Could you check a few things on this model? Use its own coordinates, in mm. A direction names the side the tool comes from. Coordinates: 2 decimals unless noted, no trailing zeros. Loops run counter-clockwise (first coordinate to the right, second up) from the corner with the lowest first, then second, coordinate; pieces in that order, holes last.
from build123d import *

# Parameters (mm, degrees)
F1_DEPTH = 25.4
F2_W     = 37.6737080514
F2_H     = 18.4638472274
F3_DEPTH = 101.6
F4_W     = 14.6301244386
F4_H     = 36.548535943
F5_DEPTH = 25.4
F6_DEPTH = 25.4
F7_W     = 18.4638472274
F7_H     = 37.6439765096
F8_DEPTH = 9.652


with BuildPart() as f1:
    # F0 (on Top) → F1 (new body)
    with BuildSketch(Plane.XY):
        with BuildLine():
            ThreePointArc((-18.8368540257, 0), (0, -18.8368540257), (18.8368540257, 0))
            Line((18.8368540257, 0), (8.9521668851, 0))
            Line((8.9521668851, 0), (-18.8368540257, 0))
        make_face()
        Polygon((-18.8368540257, 33.2889333367), (-18.8368540257, 0), (8.9521668851, 0), (8.9521668851, 14.8250861093), (18.8368540257, 14.8250861093), (18.8368540257, 33.2889333367), align=None)
    extrude(amount=F1_DEPTH)

    # F2 (on face) → F3 (join)
    with BuildSketch(Plane.XY.offset(25.4)):
        with Locations((0, 24.057009723)):
            Rectangle(F2_W, F2_H)
    extrude(amount=F3_DEPTH)

    # F4 (on face) → F5 (cut)
    with BuildSketch(Plane.XZ.offset(-14.8250861093)):
        with Locations((-0.3958076704, 108.7257320285)):
            Rectangle(F4_W, F4_H)
        with BuildLine():
            Line((6.9192545488, 90.451464057), (-7.7108698897, 90.451464057))
            ThreePointArc((-7.7108698897, 90.451464057), (-0.3958076704, 83.1364018377), (6.9192545488, 90.451464057))
        make_face()
    extrude(amount=-F5_DEPTH, mode=Mode.SUBTRACT)

    # F4 (on face) → F6 (cut)
    with BuildSketch(Plane.XZ.offset(-14.8250861093)):
        with Locations((-0.3958076704, 108.7257320285)):
            Rectangle(F4_W, F4_H)
        with BuildLine():
            Line((6.9192545488, 90.451464057), (-7.7108698897, 90.451464057))
            ThreePointArc((-7.7108698897, 90.451464057), (-0.3958076704, 83.1364018377), (6.9192545488, 90.451464057))
        make_face()
    extrude(amount=-F6_DEPTH, mode=Mode.SUBTRACT)

    # F7 (on face) → F8 (cut)
    with BuildSketch(Plane.YZ.offset(18.8368540257)):
        with Locations((24.057009723, 18.8219882548)):
            Rectangle(F7_W, F7_H)
    extrude(amount=-F8_DEPTH, mode=Mode.SUBTRACT)


solid = f1.part
(1) Imagine slicing it at A-A, the plane z = 115.5. Write out the boundary of the cut face in (x, y).
Answers:
outline: (-18.84, 14.83) - (-7.71, 14.83) - (-7.71, 33.29) - (-18.84, 33.29) - close; (6.92, 14.83) - (18.84, 14.83) - (18.84, 33.29) - (6.92, 33.29) - close
(2) We'd pull the mould along Y, two halves only. Please class faces 1 (the face through (8.952, 7, 13)), 2 (the face through (9.185, 24, 19)), 3 (the face through (0, 33.289, 63)), 4 (the face through (-0.414, -18.832, 12.522)): +Y half, -Y half, draft (parallel to the pull), parting line (faces both ways), or undercut.
Answers:
face 1: undercut
face 2: draft
face 3: +Y half
face 4: -Y half
(3) I need wall thicknesses on probe 1 along X at (y, z) = (21, 103.5); probe 2 along Z at (x, y) = (13, -7); probe 3 along Y at (x, z) = (-5, 72.5). Which ranges of each line are inside material? Lowest first, please.
Answers:
probe 1: x = -18.84 to -7.71, 6.92 to 18.84
probe 2: z = 0 to 25.4
probe 3: y = 14.83 to 33.29
(4) Imagine slicing it at D-D, the plane x = 0. Write out the boundary of the cut face in (y, z).
Answers:
outline: (-18.84, 0) - (33.29, 0) - (33.29, 83.15) - (14.83, 83.15) - (14.83, 25.4) - (-18.84, 25.4) - close
(5) Imagine slicing it at B-B, the plane z = 10. Write out the boundary of the cut face in (x, y).
Answers:
outline: (-18.84, 0) arc R18.84 ccw to (18.84, 0) - (8.95, 0) - (8.95, 14.83) - (9.18, 14.83) - (9.18, 33.29) - (-18.84, 33.29) - close
(6) Imagine slicing it at C-C, the plane y = 29. Write out the boundary of the cut face in (x, z), and give its area (3 significant figures).
Answers:
outline: (-18.84, 0) - (9.18, 0) - (9.18, 37.64) - (18.84, 37.64) - (18.84, 127) - (6.92, 127) - (6.92, 90.45) arc R7.32 cw to (-7.71, 90.45) - (-7.71, 127) - (-18.84, 127) - close
area: 3,800 mm2
(7) For pin 1 (6 mm diameter, centred on x = 5, z = 80, fed in from -Y); pin 2 (5.5 mm diameter, centred on y = 28.5, z = 23.5, fed in from +X); pin 3 (5 mm diameter, centred on x = 16, y = 28, fed in from -Z), each with a flat end and sliding along its axis, tell me the tip position at first contact or that it passes through.
Answers:
pin 1: stops at y = 14.83
pin 2: stops at x = 9.18
pin 3: stops at z = 37.64
(8) Which directions (+Z, -Z, +X, -X, +Y, -Y) give clear straight access to the entire face, cutting with the end or side of a thin tool? Please do faces 5 (the face through (14, 24, 37.644)), 6 (the face through (0, -2, 25.4)), 7 (the face through (-7.711, 24, 108)), 8 (the face through (-13, 24, 127)), 9 (the face through (-18.837, 20, 48)).
Answers:
face 5: -Z, +X, +Y, -Y
face 6: +Z, +X, -X, -Y
face 7: +Z, +Y, -Y
face 8: +Z, +X, -X, +Y, -Y
face 9: +Z, -Z, -X, +Y, -Y
